Model file for the job. Use its own axes, mm. Face numbers are marked on the shaded views. Round coordinates to 2 decimals unless told otherwise and drop trailing zeros. Order: outer loops, then holes, each group sorted by start corner. A loop starts at its lowest first (then second) coordinate and runs counter-clockwise, first axis right, second up. Notation, with made-up numbers: (17.5, -34) - (50.5, -34) arc R28 ccw to (50.5, 5) - close; hole circle Ø6 at (50, -32). An arc over 180 degrees is marked (long way). Answer as CSV lines item,"result". Start each with the question number.
1. Band-saw the part on B-B on z = 0. List the corners of the cut face in (x, y), then the cut area to 3 significant figures.
2. Pull direction X, two halves, no side cores. Call the marked faces 1, 2, 3 and 4: released by +X, released by -X, zero draft, split by the parting line, or undercut.
3. Pin check, flat tip, straight feed: pin 1 Ø5 at (x, z) = (-2.5, -2.5) entering from -Y. Stop position of the tip, or through.
4. Wall check: line 1 along X through (y, z) = (1.1, 0); line 2 along X through (y, z) = (3, -1.25); line 3 along Z through (x, y) = (0, 3.5). Give the ranges that are in metal, low to high. Write a range as [from, to].
5. Band-saw the part on A-A on y = 4.1. List the corners of the cut face in (x, z), then the cut area to 3 significant figures.
6. Band-saw the part on D-D on z = -7.25. List the corners of the cut face in (x, y), then the cut area to 3 significant figures.
7. Band-saw the part on C-C on x = 12.5. List the corners of the cut face in (y, z).
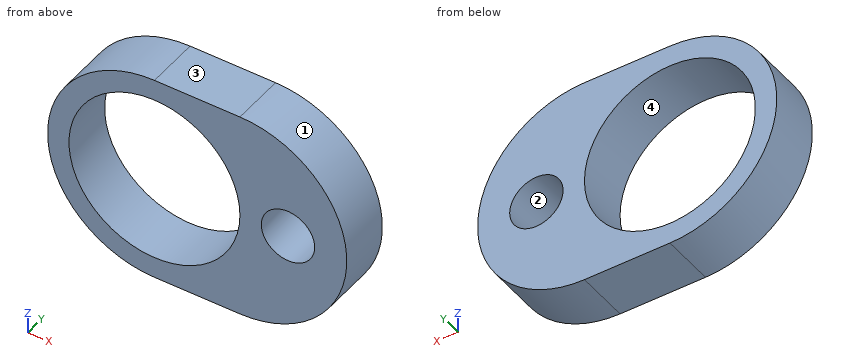
Autodesk Fusion 360 part; units mm, degrees
sketch "Boceto1" plane through (0, 0, 0) normal (0, 1, 0) x (1, 0, 0)
  circle A0 centre (0, 0) radius 10
  circle A1 centre (0, 0) radius 2.5
  circle A2 centre (0, 0) radius 8
  line L0 (0, 0) -> (12.5, 0)
  circle A3 centre (12.5, 0) radius 2.5
  line L1 (12.5, -10) -> (0, -10)
  line L2 (0, 10) -> (12.5, 10)
  circle A4 centre (8, 0) radius 10
  dimension "d1" = 5
  dimension "d5" = 16
  dimension "d7" = 12.5
extrude "Extruir1" add sketch "Boceto1" along normal blind 5 contours A0 A2 A4 | A0 L2 A4 | A0 L1 A4 | A0 A4 | A0 A2 L0 A4 | A0 A2 L0 A4
ref_plane "PlanoDeObra1" through (-10, 2.3987, 0) normal (-1, 0, 0) x (0, 0, -1)
ref_plane "PlanoDeObra2" through (18, 2.3524, 0) normal (1, 0, 0) x (0, 0, 1)
sketch "Boceto2" plane through (0, 0, 0) normal (0, -1, 0) x (1, 0, 0)
  circle A0 centre (0, 0) radius 8
  circle A1 centre (12.5, 0) radius 2.5
  arc A2 (0, 10) -> (0, -10) centre (0, 0) ccw
  line L0 (0, -10) -> (8, -10)
  arc A3 (8, -10) -> (8, 10) centre (8, 0) ccw
  line L1 (8, 10) -> (0, 10)
  circle A4 centre (12.5, 0) radius 2.5
  dimension "d11" = 5
Reply:
1,outline,"(-10, 0) - (-8, 0) - (-8, 5) - (-10, 5) - close; (8, 0) - (10, 0) - (10, 5) - (8, 5) - close; (15, 0) - (18, 0) - (18, 5) - (15, 5) - close"
1,area,"35.0 mm2"
2,face 1,"released by +X"
2,face 2,"undercut"
2,face 3,"zero draft"
2,face 4,"undercut"
3,pin 1,"passes through"
4,line 1,"x = [-10, -8], [8, 10], [15, 18]"
4,line 2,"x = [-9.92, -7.9], [7.9, 10.33], [14.67, 17.92]"
4,line 3,"z = [-10, -8], [8, 10]"
5,outline,"(0, -10) - (8, -10) arc R10 ccw to (8, 10) - (0, 10) arc R10 ccw to start; hole circle Ø16 at (0, 0); hole circle Ø5 at (12.5, 0)"
5,area,"253 mm2"
6,outline,"(-6.89, 0) - (-3.38, 0) - (-3.38, 5) - (-6.89, 5) - close; (3.38, 0) - (14.89, 0) - (14.89, 5) - (3.38, 5) - close"
6,area,"75.1 mm2"
7,outline,"(0, -8.93) - (5, -8.93) - (5, -2.5) - (0, -2.5) - close; (0, 2.5) - (5, 2.5) - (5, 8.93) - (0, 8.93) - close"
